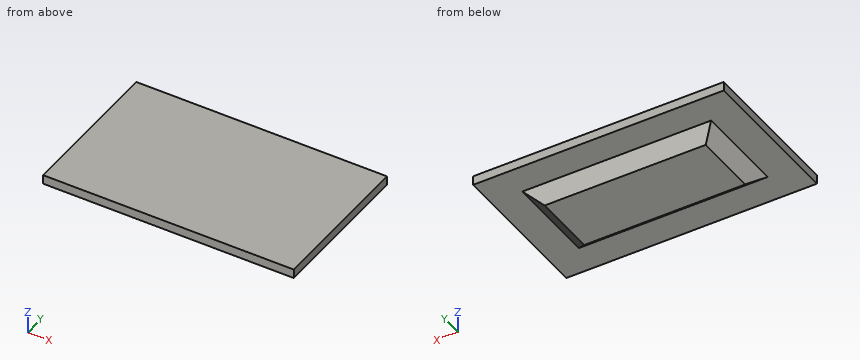
Autodesk Inventor part; units mm, degrees
ref_plane "Work Plane1" through (0, 0, -25) normal (0, 0, -1) x (-1, 0, 0)
ref_plane "YZ Plane" through (0, 0, 0) normal (1, 0, 0) x (0, 1, 0)
ref_plane "XZ Plane" through (0, 0, 0) normal (0, 1, 0) x (-1, 0, 0)
sketch "Sketch1" plane through (0, 0, 0) normal (0, 0, 1) x (1, 0, 0)
  line L0 (-272.5, -165) -> (272.5, -165)
  line L1 (272.5, -165) -> (272.5, 165)
  line L2 (272.5, 165) -> (-272.5, 165)
  line L3 (-272.5, 165) -> (-272.5, -165)
  line L4 (-272.5, -165) -> (272.5, 165) construction
  line L5 (272.5, -165) -> (-272.5, 165) construction
  point P0 (0, 0)
  dimension "d0" = 545
  dimension "d1" = 330
extrude "Extrusion1" add sketch "Sketch1" along normal blind 20
sketch "Sketch2" plane through (0, 0, 0) normal (0, 0, -1) x (-1, 0, 0)
  line L0 (-205, -100) -> (205, -100)
  line L1 (205, -100) -> (205, 100)
  line L2 (205, 100) -> (-205, 100)
  line L3 (-205, 100) -> (-205, -100)
  line L4 (-205, -100) -> (205, 100) construction
  line L5 (205, -100) -> (-205, 100) construction
  point P0 (0, 0)
  dimension "d4" = 410
  dimension "d5" = 200
ref_plane "Work Plane1" through (0, 0, -25) normal (0, 0, -1) x (-1, 0, 0)
sketch "Sketch3" plane through (0, 0, -25) normal (0, 0, -1) x (-1, 0, 0)
  line L0 (-175, -70) -> (175, -70)
  line L1 (175, -70) -> (175, 70)
  line L2 (175, 70) -> (-175, 70)
  line L3 (-175, 70) -> (-175, -70)
  line L4 (-175, -70) -> (175, 70) construction
  line L5 (175, -70) -> (-175, 70) construction
  point P0 (0, 0)
  dimension "d7" = 350
  dimension "d8" = 140
loft "Loft1" add profiles "Sketch2", "Sketch3"
properties part number "ShedMonitor"
For this review, take the finished solid that the model builds, in its own axes (mm). Round coordinates to 2 decimals unless told otherwise and drop trailing zeros. Loops run counter-clockwise (first coordinate to the right, second up) from the corner with the lowest first, then second, coordinate; pieces in that order, holes last. Notation, with made-up numbers: (70, 43.25) - (104, 43.25) arc R21 cw to (104, 49.25) - close; hole circle Ø2 at (73.5, 77). An arc over 180 degrees is marked (long way). Use one line per item in the form item = value.
1) We need section A-A on x = 211. Write out the cut boundary in (y, z).
Solutions:
outline = (-165, 0) - (165, 0) - (165, 20) - (-165, 20) - close
2) Clearance check with flat-ended pins moving along their axes: P1, Ø12, axis at x = -135.5, y = 131, coming from the -Z side; P2, Ø2, axis at x = 139.5, z = -18.5, coming from the -Y side; P3, Ø10, axis at x = 127.5, y = 80, coming from the -Z side; P4, Ø6, axis at x = -76, y = 71, coming from the -Z side. State where each tip first meets the part, or that it passes through.
Solutions:
P1 = 0
P2 = -79
P3 = -20.83
P4 = -25
3) Wall thickness on probe 1 along Z at (x, y) = (213, 78.5); probe 2 along Y at (x, z) = (-57, -4); probe 3 along X at (y, z) = (42, -10): over which ranges is each line inside the solid? List them lowest first.
Solutions:
probe_1 = 0 to 20
probe_2 = -95.2 to 95.2
probe_3 = -193 to 193
4) We need section B-B on y = 138.5. Write out the cut boundary in (x, z), then the cut area to 3 significant figures.
Solutions:
outline = (-272.5, 0) - (272.5, 0) - (272.5, 20) - (-272.5, 20) - close
area = 10,900 mm2
